For this review, take the finished solid that the model builds, in its own axes (mm). Give positions to 0.01 mm unless a question says otherwise; leave off trailing zeros. Order: outer loops, then holes, each group sorted by start corner. A loop starts at its lowest first (then second) coordinate and runs counter-clockwise, first axis right, second up.
from build123d import *

# Parameters (mm, degrees)
SKIZZE1_W                       = 40
SKIZZE1_H                       = 20
SKIZZE1_W_2                     = 36
SKIZZE1_H_2                     = 16
AUFSATZ_LINEAR_AUSTRAGEN1_DEPTH = 220
SKIZZE2_R                       = 1.7
SCHNITT_LINEAR_AUSTRAGEN1_DEPTH = 222.810730128
SKIZZE4_R                       = 3.7
SCHNITT_LINEAR_AUSTRAGEN2_DEPTH = 5
SKIZZE2_3_R                     = 4.5
SCHNITT_LINEAR_AUSTRAGEN3_DEPTH = 5


with BuildPart() as part:
    # Skizze1 → Aufsatz-Linear austragen1 (new body)
    with BuildSketch(Plane(origin=(0, 0, 0), x_dir=(0, 0, -1), z_dir=(1, 0, 0))):
        Rectangle(SKIZZE1_W, SKIZZE1_H)
        Rectangle(SKIZZE1_W_2, SKIZZE1_H_2, mode=Mode.SUBTRACT)
    extrude(amount=AUFSATZ_LINEAR_AUSTRAGEN1_DEPTH)

    # Skizze2 → Schnitt-Linear austragen1 (cut, through all)
    with BuildSketch(Plane(origin=(0, 10, 0), x_dir=(1, 0, 0), z_dir=(0, 1, 0))):
        with BuildLine():
            Line((20, 20), (0, 20))
            Line((0, 20), (0, -4.7e-08))
            ThreePointArc((0, -4.7e-08), (5.85786436, 14.142135607), (20, 20))
        make_face()
        with BuildLine():
            ThreePointArc((20, -20), (5.857864393, -14.14213564), (0, -4.7e-08))
            Line((0, -4.7e-08), (0, -20))
            Line((0, -20), (20, -20))
        make_face()
        with BuildLine():
            Line((220, 20), (200, 20))
            ThreePointArc((200, 20), (214.142135624, 14.142135624), (220, 0))
            Line((220, 0), (220, 20))
        make_face()
        with BuildLine():
            ThreePointArc((220, 0), (214.142135624, -14.142135624), (200, -20))
            Line((200, -20), (220, -20))
            Line((220, -20), (220, 0))
        make_face()
        with Locations(Location((30.25, 0, 0), (0, 0, 270))):
            Circle(SKIZZE2_R)
        with Locations(Location((189.75, 0, 0), (0, 0, 270))):
            Circle(SKIZZE2_R)
        with Locations(Location((25.125, -8.876760389, 0), (0, 0, 270))):
            Circle(SKIZZE2_R)
        with Locations(Location((14.875, -8.876760389, 0), (0, 0, 270))):
            Circle(SKIZZE2_R)
        with Locations(Location((9.75, 0, 0), (0, 0, 270))):
            Circle(SKIZZE2_R)
        with Locations(Location((14.875, 8.876760389, 0), (0, 0, 270))):
            Circle(SKIZZE2_R)
        with Locations(Location((25.125, 8.876760389, 0), (0, 0, 270))):
            Circle(SKIZZE2_R)
        with Locations(Location((194.875, 8.876760389, 0), (0, 0, 270))):
            Circle(SKIZZE2_R)
        with Locations(Location((205.125, 8.876760389, 0), (0, 0, 270))):
            Circle(SKIZZE2_R)
        with Locations(Location((210.25, 0, 0), (0, 0, 270))):
            Circle(SKIZZE2_R)
        with Locations(Location((205.125, -8.876760389, 0), (0, 0, 270))):
            Circle(SKIZZE2_R)
        with Locations(Location((194.875, -8.876760389, 0), (0, 0, 270))):
            Circle(SKIZZE2_R)
    extrude(amount=-SCHNITT_LINEAR_AUSTRAGEN1_DEPTH, mode=Mode.SUBTRACT)

    # Skizze4 → Schnitt-Linear austragen2 (cut)
    with BuildSketch(Plane.XZ.offset(10)):
        with Locations(Location((189.75, 0, 0), (0, 0, 270))):
            Circle(SKIZZE4_R)
        with Locations(Location((194.875, -8.876760389, 0), (0, 0, 270))):
            Circle(SKIZZE4_R)
        with Locations(Location((205.125, -8.876760389, 0), (0, 0, 270))):
            Circle(SKIZZE4_R)
        with Locations(Location((210.25, 0, 0), (0, 0, 270))):
            Circle(SKIZZE4_R)
        with Locations(Location((205.125, 8.876760389, 0), (0, 0, 270))):
            Circle(SKIZZE4_R)
        with Locations(Location((194.875, 8.876760389, 0), (0, 0, 270))):
            Circle(SKIZZE4_R)
        with Locations(Location((30.25, 0, 0), (0, 0, 270))):
            Circle(SKIZZE4_R)
        with Locations(Location((25.125, -8.876760389, 0), (0, 0, 270))):
            Circle(SKIZZE4_R)
        with Locations(Location((14.875, -8.876760389, 0), (0, 0, 270))):
            Circle(SKIZZE4_R)
        with Locations(Location((9.75, 0, 0), (0, 0, 270))):
            Circle(SKIZZE4_R)
        with Locations(Location((25.125, 8.876760389, 0), (0, 0, 270))):
            Circle(SKIZZE4_R)
        with Locations(Location((14.875, 8.876760389, 0), (0, 0, 270))):
            Circle(SKIZZE4_R)
    extrude(amount=-SCHNITT_LINEAR_AUSTRAGEN2_DEPTH, mode=Mode.SUBTRACT)

    # Skizze2_3 → Schnitt-Linear austragen3 (cut)
    with BuildSketch(Plane(origin=(0, 10, 0), x_dir=(1, 0, 0), z_dir=(0, 1, 0))):
        with Locations(Location((20, 0, 0), (0, 0, 270))):
            Circle(SKIZZE2_3_R)
        with Locations(Location((200, 0, 0), (0, 0, 270))):
            Circle(SKIZZE2_3_R)
    extrude(amount=-SCHNITT_LINEAR_AUSTRAGEN3_DEPTH, mode=Mode.SUBTRACT)


solid = part.part
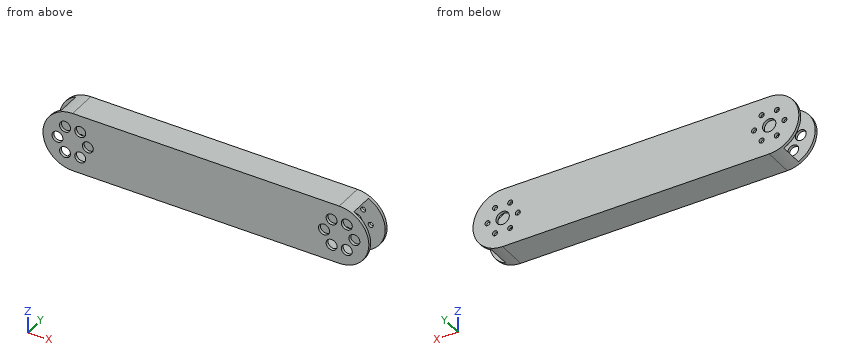
1) Clearance check with flat-ended pins moving along their axes: pin 1 (1.5 mm diameter, centred on y = 7, z = 13.5, fed in from +X); pin 2 (6 mm diameter, centred on x = 194.88, z = -8.88, fed in from -Y). State where each tip first meets the part, or that it passes through.
Answer sheet:
pin 1: passes through
pin 2: stops at y = 8
2) We need section A-A on x = 129. Give the boundary of the cut face in (y, z), then the cut area to 3 significant figures.
Answer sheet:
outline: (-10, -20) - (10, -20) - (10, 20) - (-10, 20) - close; hole (-8, -18) - (8, -18) - (8, 18) - (-8, 18) - close
area: 224 mm2
3) To check wall thickness, follow line 1 (Y direction, x = 123, z = -4.5); line 2 (Z direction, x = 81, y = 7); line 3 (Z direction, x = 210.25, y = 8.5). State the ranges of each line that lie inside material, in increasing order.
Answer sheet:
line 1: y = -10 to -8, 8 to 10
line 2: z = -20 to -18, 18 to 20
line 3: z = -17.17 to -1.7, 1.7 to 17.17
4) We need section B-B on y = 1.5. Give the boundary of the cut face in (x, z), then the cut area to 3 significant figures.
Answer sheet:
outline: (11.28, -18) arc R20 ccw to (20, -20) - (200, -20) arc R20 ccw to (208.72, -18) - close; (11.28, 18) - (208.72, 18) arc R20 ccw to (200, 20) - (20, 20) arc R20 ccw to start
area: 767 mm2
